from build123d import *

# Parameters (mm, degrees)
SKETCH1_R                                = 125.73
SKETCH1_R_2                              = 50.8
EXTRUDE1_DEPTH                           = 1.524
F_5_16_CLEARANCE_HOLE1_D                 = 8.4328
CIRPATTERN1_COUNT                        = 3
F_1_4_20_WELD_NUT_CIRPATTERN_COUNT       = 3
HOLE_FOR_5_16_18_WELD_NUT_D              = 15.9766
HOLE_FOR_5_16_18_WELD_NUT_DEPTH          = 21.59
F_5_16_18_WELD_NUT_HOLE_CIRPATTERN_COUNT = 3
CHAMFER4_SIZE                            = 0.635
F_6_CLEARANCE_HOLE1_D                    = 4.3053
CIRPATTERN2_COUNT                        = 4
CIRPATTERN3_COUNT                        = 3
CIRPATTERN3_COPY_1_D                     = 4.3053
CIRPATTERN3_COPY_2_D                     = 4.3053
CIRPATTERN3_COPY_3_D                     = 4.3053
CIRPATTERN3_COPY_4_D                     = 4.3053
CIRPATTERN3_COPY_5_D                     = 4.3053
CIRPATTERN3_COPY_6_D                     = 4.3053


with BuildPart() as part:
    # Sketch1 → Extrude1 (new body)
    with BuildSketch(Plane(origin=(0, 0, 0), x_dir=(1, 0, 0), z_dir=(0, 1, 0))):
        with Locations(Location((0, 0, 0), (0, 0, 270))):  # turned: the seam where the file's is
            Circle(SKETCH1_R)
        with Locations(Location((0, 0, 0), (0, 0, 270))):  # turned: the seam where the file's is
            Circle(SKETCH1_R_2, mode=Mode.SUBTRACT)
    extrude(amount=EXTRUDE1_DEPTH)

    # 5_16 Clearance Hole1 (through all)
    with Locations(Plane(origin=(0, 1.524, 0), x_dir=(-1, 0, 0), z_dir=(0, 1, 0))):
        with Locations((0, 115.9256)):
            f_5_16_clearance_hole1 = Hole(F_5_16_CLEARANCE_HOLE1_D / 2)

    # CirPattern1: 5_16 Clearance Hole1 ×3 about axis
    cirpattern1_axis = Axis((0, 0, 0), (0, 1, 0))
    for i in range(1, CIRPATTERN1_COUNT):
        add(f_5_16_clearance_hole1.rotate(cirpattern1_axis, i * 360 / CIRPATTERN1_COUNT), mode=Mode.SUBTRACT)

    # Sketch4 → Hole For 1_4_-20 Weld Nut (revolve, cut)
    with BuildSketch(Plane(origin=(0, 1.524, -76.2), x_dir=(0, 0, 1), z_dir=(1, 0, 0))):
        Polygon((0, 0), (0, 16.54598865), (6.4008, 12.7), (6.4008, 0), align=None)
    hole_for_1_4_20_weld_nut = revolve(axis=Axis((0, 7.874, -76.2), (0, -1, 0)), mode=Mode.SUBTRACT)

    # 1_4_-20 Weld Nut CirPattern: Hole For 1_4_-20 Weld Nut ×3 about axis
    f_1_4_20_weld_nut_cirpattern_axis = Axis((0, 0, 0), (0, 1, 0))
    for i in range(1, F_1_4_20_WELD_NUT_CIRPATTERN_COUNT):
        add(hole_for_1_4_20_weld_nut.rotate(f_1_4_20_weld_nut_cirpattern_axis, i * 360 / F_1_4_20_WELD_NUT_CIRPATTERN_COUNT), mode=Mode.SUBTRACT)

    # Hole For 5_16_-18 Weld Nut
    with Locations(Plane(origin=(0, 1.524, 0), x_dir=(-1, 0, 0), z_dir=(0, 1, 0))):
        with Locations((0, -76.2)):
            hole_for_5_16_18_weld_nut = Hole(HOLE_FOR_5_16_18_WELD_NUT_D / 2, depth=HOLE_FOR_5_16_18_WELD_NUT_DEPTH)

    # 5_16_-18 Weld Nut Hole CirPattern: Hole For 5_16_-18 Weld Nut ×3 about axis
    f_5_16_18_weld_nut_hole_cirpattern_axis = Axis((0, 0, 0), (0, 1, 0))
    for i in range(1, F_5_16_18_WELD_NUT_HOLE_CIRPATTERN_COUNT):
        add(hole_for_5_16_18_weld_nut.rotate(f_5_16_18_weld_nut_hole_cirpattern_axis, i * 360 / F_5_16_18_WELD_NUT_HOLE_CIRPATTERN_COUNT), mode=Mode.SUBTRACT)

    # Chamfer4
    chamfer4_edges = [part.edges().sort_by_distance(p)[0] for p in [
        (-7.9883, 0, -76.2),
        (69.985285768, 0, 31.181929267),
        (-61.996985768, 0, 45.018070733),
    ]]
    chamfer(chamfer4_edges, length=CHAMFER4_SIZE)

    # 6 Clearance Hole1 (through all)
    with Locations(Plane.XZ):
        with Locations((-54.99261314, 31.75)):
            f_6_clearance_hole1 = Hole(F_6_CLEARANCE_HOLE1_D / 2)

    # CirPattern2: 6 Clearance Hole1 ×4 about axis
    cirpattern2_axis = Axis((-65.991135768, 0, 38.1), (0, 1, 0))
    for i in range(1, CIRPATTERN2_COUNT):
        add(f_6_clearance_hole1.rotate(cirpattern2_axis, i * 360 / CIRPATTERN2_COUNT), mode=Mode.SUBTRACT)

    # CirPattern3: 6 Clearance Hole1 ×3 about axis
    cirpattern3_axis = Axis((0, 0, 0), (0, 1, 0))
    for i in range(1, CIRPATTERN3_COUNT):
        add(f_6_clearance_hole1.rotate(cirpattern3_axis, i * 360 / CIRPATTERN3_COUNT), mode=Mode.SUBTRACT)

    # CirPattern3 copy 1 (through all)
    with Locations(Plane(origin=(27.891135768, 0, 104.091135768), x_dir=(-0.866025404, 0, 0.5), z_dir=(0, -1, 0))):
        with Locations((-54.99261314, 31.75)):
            Hole(CIRPATTERN3_COPY_1_D / 2)

    # CirPattern3 copy 2 (through all)
    with Locations(Plane(origin=(76.2, 0, -76.2), x_dir=(0.866025404, 0, 0.5), z_dir=(0, -1, 0))):
        with Locations((-54.99261314, 31.75)):
            Hole(CIRPATTERN3_COPY_2_D / 2)

    # CirPattern3 copy 3 (through all)
    with Locations(Plane(origin=(131.982271537, 0, 76.2), x_dir=(0.5, 0, 0.866025404), z_dir=(0, -1, 0))):
        with Locations((-54.99261314, 31.75)):
            Hole(CIRPATTERN3_COPY_3_D / 2)

    # CirPattern3 copy 4 (through all)
    with Locations(Plane(origin=(0, 0, -152.4), x_dir=(0.5, 0, -0.866025404), z_dir=(0, -1, 0))):
        with Locations((-54.99261314, 31.75)):
            Hole(CIRPATTERN3_COPY_4_D / 2)

    # CirPattern3 copy 5 (through all)
    with Locations(Plane(origin=(104.091135768, 0, -27.891135768), x_dir=(0.866025404, 0, -0.5), z_dir=(0, -1, 0))):
        with Locations((-54.99261314, 31.75)):
            Hole(CIRPATTERN3_COPY_5_D / 2)

    # CirPattern3 copy 6 (through all)
    with Locations(Plane(origin=(-76.2, 0, -76.2), x_dir=(-0.866025404, 0, -0.5), z_dir=(0, -1, 0))):
        with Locations((-54.99261314, 31.75)):
            Hole(CIRPATTERN3_COPY_6_D / 2)


solid = part.part
Verification items for the finished model (mm, model axes). Give positions to 0.01 mm unless a question says otherwise; leave off trailing zeros. Order: outer loops, then holes, each group sorted by start corner. A loop starts at its lowest first (then second) coordinate and runs counter-clockwise, first axis right, second up. Notation, with made-up numbers: M 30.25,-38.5 L 66.25,-38.5 A15 ccw 66.25,-20.5 Z; hole C 44,-12.5 d8. An arc over 180 degrees is marked long. Answer as a JSON object with one key per item and string values. Group by question number.
1) Cross-section at D-D (z = 74.5). Enter the section's corners in (x, y), then the cut area to 3 significant figures.
2) Mould release check, pull along X, two halves, no side actions. Record for faces 1 (the face through (-76.5, 0.75, -99.78)), 2 (the face through (-62.31, 1.07, 31.01)), 3 (the face through (-54, 0, -2)): released by +X, released by -X, zero draft, split by the parting line, or undercut.
3) Cross-section at B-B (y = 0.3). Give the number of separate pieces and of enclosed holes in the cut face, then the cut area to 3 significant figures.
4) Cross-section at C-C (x = -47). Enter the section's corners in (y, z).
5) Cross-section at A-A (z = -31). Enter the section's corners in (x, y).
6) Scan lines: line 1 along X through (y, z) = (0.45, 36.5); line 2 along Z through (x, y) = (-13, 0.6); line 3 along X through (y, z) = (0.5, -76.2). Record each from-to range of solid material in increasing order. Write a range as [from, to].
Result sheet:
{
 "1": {"outline": "M -101.28,0 L 101.28,0 L 101.28,1.52 L -101.28,1.52 Z", "area": "309 mm2"},
 "2": {"face 1": "split by the parting line", "face 2": "undercut", "face 3": "zero draft"},
 "3": {"separate pieces": "1", "enclosed holes": "19", "area": "40,600 mm2"},
 "4": {"outline": "M 0,-116.61 L 1.52,-116.61 L 1.52,-19.28 L 0,-19.28 Z; M 0,19.28 L 1.52,19.28 L 1.52,116.61 L 0,116.61 Z"},
 "5": {"outline": "M -121.85,0 L -40.24,0 L -40.24,1.52 L -121.85,1.52 Z; M 40.24,0 L 121.85,0 L 121.85,1.52 L 40.24,1.52 Z"},
 "6": {"line 1": "x = [-120.32, -74.01], [-57.98, -35.33], [35.33, 57.98], [74.01, 120.32]", "line 2": "z = [-125.06, -78.33], [-74.07, -49.11], [49.11, 125.06]", "line 3": "x = [-100.01, -14.85], [-10.55, -8.12], [8.12, 10.55], [14.85, 100.01]"}
}
